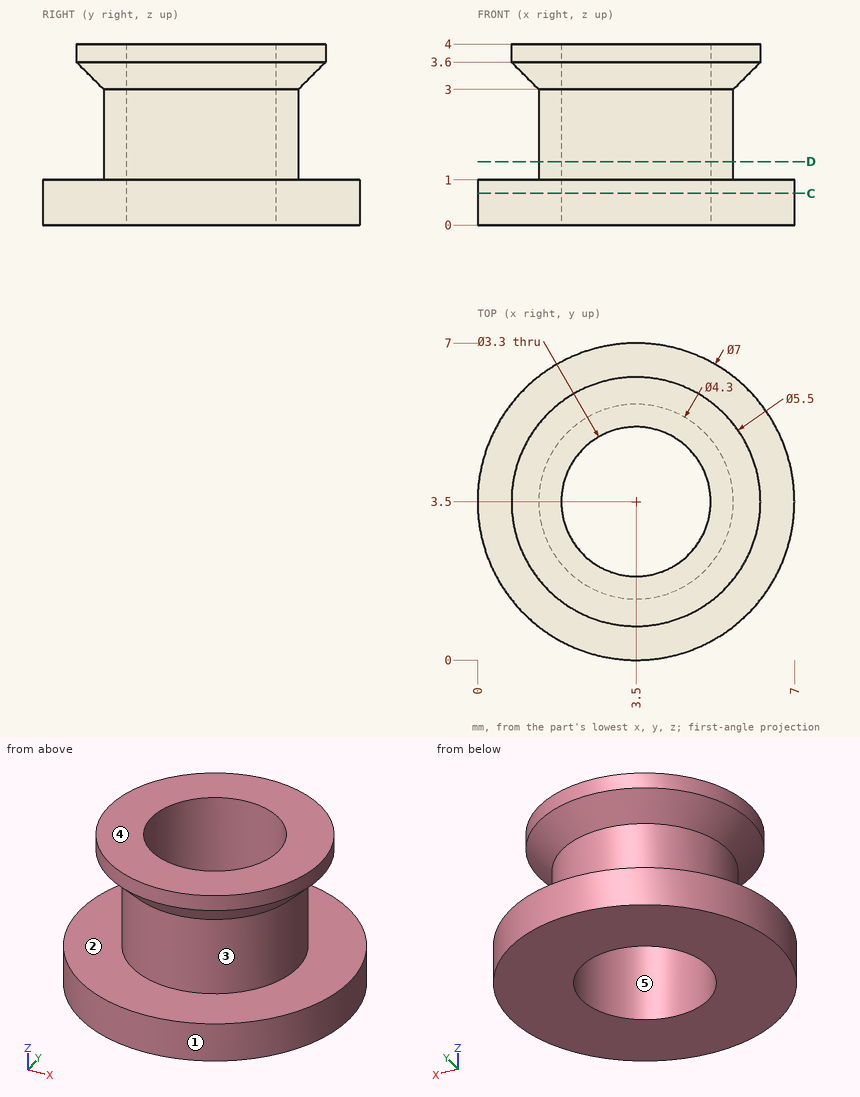
Check sheet for the drawn part. Datum: minimum x, y, z corner. Units: mm. A direction names the side the tool comes from. Round coordinates to 2 decimals unless told otherwise and drop trailing zeros. Loops run counter-clockwise (first coordinate to the right, second up) from the corner with the lowest first, then second, coordinate; pieces in that order, holes last. Notation, with made-up numbers: (-25, -15.5) - (21, -15.5) arc R3 cw to (21, -10.5) - close; hole circle Ø2 at (-40, -17). An arc over 180 degrees is marked (long way). Write each question's results on one line, items separated by ' | '. Start each with the question number.
Q1. Thickness scan on line 1 (Y direction, x = 3.5, z = 2.85); line 2 (Z direction, x = 5.5, y = 5.75); line 3 (X direction, y = 2, z = 3.25). Record the ranges inside material, lowest first. Write a range as [from, to].
Q2. Cross-section at D-D on z = 1.4. Enter the section's corners in (x, y).
Q3. Cross-section at C-C on z = 0.7. Enter the section's corners in (x, y), and give its area (3 significant figures).
Q4. Release check for a two-part mould opening along X. For the marked faces 3, 4 and 5 record: +X half, -X half, draft (parallel to the pull), parting line (faces both ways), or undercut.
Q5. Gauge pin test, flat end, axial feed: P1, Ø2, axis at y = 1, z = 3, coming from the -X side. Record the tip position at first contact, or that the pin passes through.
Q6. Access from +Z, -Z, +X, -X, +Y, -Y to the whole of each face (thin tool, end or side, straight path). Record for the marked faces 1 and 2.
Answers below:
1) line 1: y = [1.35, 1.85], [5.15, 5.65] | line 2: z = [0, 1] | line 3: x = [1.63, 2.81], [4.19, 5.37]
2) outline: circle Ø4.3 at (3.5, 3.5); hole circle Ø3.3 at (3.5, 3.5)
3) outline: circle Ø7 at (3.5, 3.5); hole circle Ø3.3 at (3.5, 3.5) | area: 29.9 mm²
4) face 3: parting line | face 4: draft | face 5: undercut
5) P1: stops at x = 1.34
6) face 1: +Z, -Z | face 2: none
